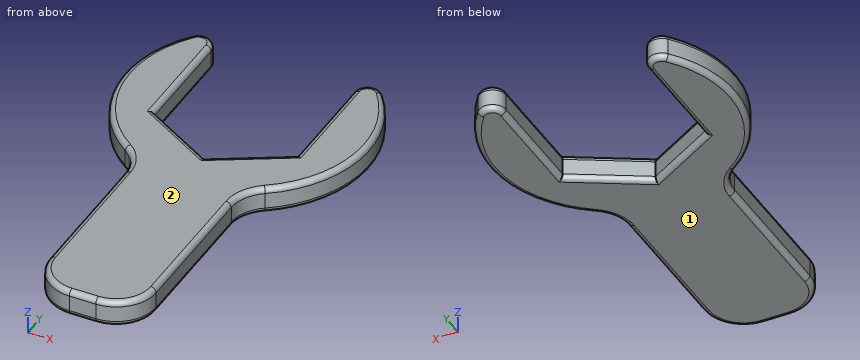
from build123d import *

# Parameters (mm, degrees)
F1_DEPTH = 6.35
F2_R     = 1.27


with BuildPart() as f1:
    # F0 (on Top) → F1 (new body)
    with BuildSketch(Plane.XY):
        with BuildLine():
            Line((17.145, 16.455425), (17.145, 9.89867))
            Line((17.145, 9.89867), (17.145, -9.89867))
            Line((17.145, -9.89867), (0, -19.797341))
            Line((0, -19.797341), (-17.145, -9.89867))
            Line((-17.145, -9.89867), (-17.145, 9.89867))
            Line((-17.145, 9.89867), (-17.145, 16.455425))
            ThreePointArc((-17.145, 16.455425), (-19.260136, 19.448303), (-22.787402, 18.453563))
            ThreePointArc((-22.787402, 18.453563), (-29.033356, -4.106567), (-16.775641, -24.049481))
            ThreePointArc((-16.775641, -24.049481), (-13.780156, -27.455953), (-12.7, -31.861658))
            Line((-12.7, -31.861658), (-12.7, -66.675))
            ThreePointArc((-12.7, -66.675), (-9.910192, -73.410192), (-3.175, -76.2))
            Line((-3.175, -76.2), (3.175, -76.2))
            ThreePointArc((3.175, -76.2), (9.910192, -73.410192), (12.7, -66.675))
            Line((12.7, -66.675), (12.7, -31.861658))
            ThreePointArc((12.7, -31.861658), (13.780156, -27.455953), (16.775641, -24.049481))
            ThreePointArc((16.775641, -24.049481), (29.033356, -4.106567), (22.787402, 18.453563))
            ThreePointArc((22.787402, 18.453563), (19.260136, 19.448303), (17.145, 16.455425))
        make_face()
    extrude(amount=F1_DEPTH)

    # F2
    f2_edges = [f1.edges().sort_by_distance(p)[0] for p in [
        (-13.780156, -27.455953, 6.35),
        (-12.7, -49.268329, 6.35),
        (-9.910192, -73.410192, 6.35),
        (0, -76.2, 6.35),
        (9.910192, -73.410192, 6.35),
        (12.7, -49.268329, 6.35),
        (13.780156, -27.455953, 6.35),
        (29.033356, -4.106567, 6.35),
        (19.260136, 19.448303, 6.35),
        (17.145, 3.278378, 6.35),
        (8.5725, -14.848006, 6.35),
        (-8.5725, -14.848006, 6.35),
        (-17.145, 3.278378, 6.35),
        (-19.260136, 19.448303, 6.35),
        (-29.033356, -4.106567, 6.35),
        (-13.780156, -27.455953, 0),
        (-12.7, -49.268329, 0),
        (-9.910192, -73.410192, 0),
        (0, -76.2, 0),
        (9.910192, -73.410192, 0),
        (12.7, -49.268329, 0),
        (13.780156, -27.455953, 0),
        (29.033356, -4.106567, 0),
        (19.260136, 19.448303, 0),
        (17.145, 3.278378, 0),
        (8.5725, -14.848006, 0),
        (-8.5725, -14.848006, 0),
        (-17.145, 3.278378, 0),
        (-19.260136, 19.448303, 0),
        (-29.033356, -4.106567, 0),
    ]]
    fillet(f2_edges, radius=F2_R)


solid = f1.part
Geometry check sheet. Reference: the model listing, model coordinates, mm. Face numbers are marked on the shaded views. Give positions to 0.01 mm unless a question says otherwise; leave off trailing zeros. Order: outer loops, then holes, each group sorted by start corner. A loop starts at its lowest first (then second) coordinate and runs counter-clockwise, first axis right, second up.
1) Material ranges on probe 1 along X at (y, z) = (-32, 2.75); probe 2 along X at (y, z) = (9, 1); probe 3 along X at (y, z) = (-18, 2.75), recorded low to high.
Results are:
probe 1: x = -12.7 to 12.7
probe 2: x = -27.88 to -17.17, 17.17 to 27.88
probe 3: x = -23.15 to -3.11, 3.11 to 23.15
2) Cross-section at B-B (y = -47). Record the boundary of the cut face in (x, z).
Results are:
outline: (-12.7, 1.27) arc R1.27 ccw to (-11.43, 0) - (11.43, 0) arc R1.27 ccw to (12.7, 1.27) - (12.7, 5.08) arc R1.27 ccw to (11.43, 6.35) - (-11.43, 6.35) arc R1.27 ccw to (-12.7, 5.08) - close
3) Cross-section at A-A (z = 3.5). Record the boundary of the cut face in (x, y) (3 decimals), then the cut area to 3 significant figures.
Results are:
outline: (-22.787, 18.454) arc R29.322 ccw to (-16.776, -24.049) arc R9.525 cw to (-12.7, -31.862) - (-12.7, -66.675) arc R9.525 ccw to (-3.175, -76.2) - (3.175, -76.2) arc R9.525 ccw to (12.7, -66.675) - (12.7, -31.862) arc R9.525 cw to (16.776, -24.049) arc R29.322 ccw to (22.787, 18.454) arc R3.175 ccw to (17.145, 16.455) - (17.145, -9.899) - (0, -19.797) - (-17.145, -9.899) - (-17.145, 16.455) arc R3.175 ccw to start
area: 2,410 mm2
4) Draft check along Z on the marked faces 1 and 2. Enter one of: released by +Z, released by -Z, zero draft, split by the parting line, or undercut.
Results are:
face 1: released by -Z
face 2: released by +Z
5) Gauge pin test, flat ends, axial feed: pin 1 (1 mm diameter, centred on y = -19.5, z = 5.5, fed in from -X); pin 2 (1 mm diameter, centred on y = -18, z = 4, fed in from -X); pin 3 (1.5 mm diameter, centred on y = 9.5, z = 2.5, fed in from +X); pin 4 (6 mm diameter, centred on x = -16.5, y = -11.5, fed in from +Z). Record the tip position at first contact, or that the pin passes through.
Results are:
pin 1: stops at x = -22.28
pin 2: stops at x = -23.53
pin 3: stops at x = 27.99
pin 4: stops at z = 6.35
